Geometry: see drawing. Coordinates: mm, zero at the bounding-box minimum. Give positions to 0.01 mm unless a question says otherwise; leave off trailing zeros. Write each loop counter-clockwise with the first axis right and the second up, starting at its lowest first coordinate (ties: lowest second). Pieces come first, ordered by that corner, then holes.
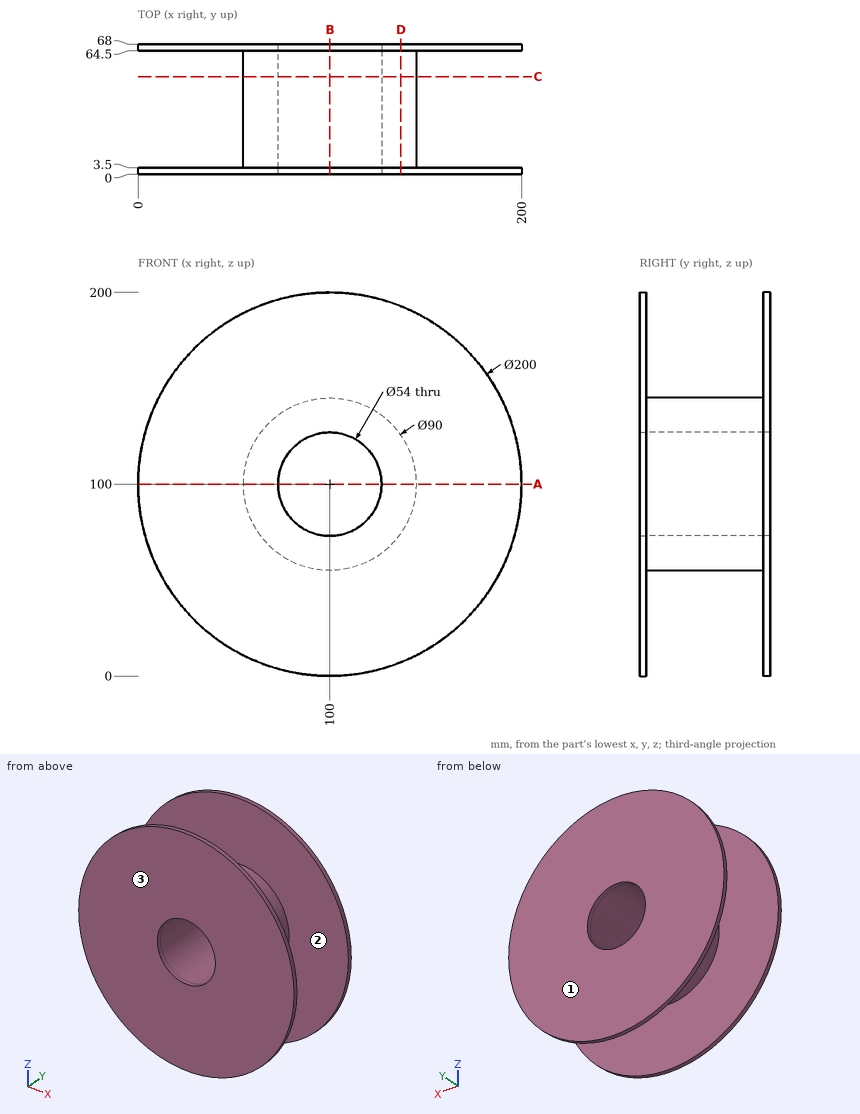
1. Section query B-B (x = 100). Return loops of the section in (y, z), plus the area to 3 significant figures.
2. Section query C-C (y = 51). Return loops of the section in (x, z).
3. Line query: probe 1 along Y at (x, z) = (83.5, 11); probe 2 along Z at (x, y) = (100, 48.5); probe 3 along Z at (x, y) = (100, 2). Output: solid intervals per line, ascending.
4. Section query D-D (x = 137). Return loops of the section in (y, z).
5. Pin query (flat end, axial travel): P1, Ø10, axis at x = 122, y = 54.5, coming from the -Z side; P2, Ø8, axis at x = 31.5, z = 174, coming from the +Y side; P3, Ø1.5, axis at x = 86, y = 17, coming from the -Z side; P4, Ø1.5, axis at x = 108, y = 17.5, coming from the +Z side. Return the tip coordinate at first contact, or that it passes through.
6. Section query A-A (z = 100). Return loops of the section in (x, y).
7. Pull-direction query (Y, two-part tool) for the marked faces 1, 2 and 3; classes: pulls with the +Y half, pulls with the -Y half, needs draft (parallel to the pull), parting line crosses it, or undercut.
The answers:
1. outline: (0, 0) - (3.5, 0) - (3.5, 55) - (64.5, 55) - (64.5, 0) - (68, 0) - (68, 73) - (0, 73) - close; (0, 127) - (68, 127) - (68, 200) - (64.5, 200) - (64.5, 145) - (3.5, 145) - (3.5, 200) - (0, 200) - close
1. area: 3,220 mm2
2. outline: circle Ø90 at (100, 100); hole circle Ø54 at (100, 100)
3. probe 1: y = 0 to 3.5, 64.5 to 68
3. probe 2: z = 55 to 73, 127 to 145
3. probe 3: z = 0 to 73, 127 to 200
4. outline: (0, 7.1) - (3.5, 7.1) - (3.5, 74.39) - (64.5, 74.39) - (64.5, 7.1) - (68, 7.1) - (68, 192.9) - (64.5, 192.9) - (64.5, 125.61) - (3.5, 125.61) - (3.5, 192.9) - (0, 192.9) - close
5. P1: stops at z = 58.33
5. P2: stops at y = 68
5. P3: stops at z = 56.99
5. P4: stops at z = 144.41
6. outline: (0, 0) - (73, 0) - (73, 68) - (0, 68) - (0, 64.5) - (55, 64.5) - (55, 3.5) - (0, 3.5) - close; (127, 0) - (200, 0) - (200, 3.5) - (145, 3.5) - (145, 64.5) - (200, 64.5) - (200, 68) - (127, 68) - close
7. face 1: pulls with the +Y half
7. face 2: undercut
7. face 3: pulls with the -Y half
